```python
from build123d import *

# Parameters (mm, degrees)
SKETCH1_W                = 44.45
SKETCH1_H                = 57.15
SKETCH1_R                = 1.5875
BOSS_EXTRUDE1_DEPTH      = 1.5875
BOSS_EXTRUDE2_DEPTH      = 11.43
BOSS_EXTRUDE2_DEPTH_BACK = 3.81
BOSS_EXTRUDE3_REACH      = 120.467


with BuildPart() as part:
    # Sketch1 → Boss-Extrude1 (new body)
    with BuildSketch(Plane(origin=(0, 0, 0), x_dir=(1, 0, 0), z_dir=(0, 1, 0))):
        with Locations((-61.695053498, -38.539128831)):
            Rectangle(SKETCH1_W, SKETCH1_H)
        with Locations(Location((-80.745053498, -63.939128831, 0), (0, 0, 270))):
            Circle(SKETCH1_R, mode=Mode.SUBTRACT)
        with Locations(Location((-42.645053498, -63.939128831, 0), (0, 0, 270))):
            Circle(SKETCH1_R, mode=Mode.SUBTRACT)
        with Locations(Location((-42.645053498, -13.139128831, 0), (0, 0, 270))):
            Circle(SKETCH1_R, mode=Mode.SUBTRACT)
        with Locations(Location((-80.745053498, -13.139128831, 0), (0, 0, 270))):
            Circle(SKETCH1_R, mode=Mode.SUBTRACT)
    extrude(amount=BOSS_EXTRUDE1_DEPTH)

    # Sketch2 → Boss-Extrude2 (add, two sides: drawn at the far end of the back side and taken through both)
    with BuildSketch(Plane(origin=(0, 1.5875, 0), x_dir=(1, 0, 0), z_dir=(0, 1, 0)).offset(-BOSS_EXTRUDE2_DEPTH_BACK)):
        Polygon((-99.160053498, -6.789128831), (-83.920053498, -6.789128831), (-83.920053498, -70.289128831), (-99.160053498, -70.289128831), (-99.160053498, -69.394762634), (-86.755200336, -69.394762634), (-86.755200336, -64.028565451), (-99.160053498, -64.028565451), (-99.160053498, -63.134199254), (-86.755200336, -63.134199254), (-86.755200336, -57.768002071), (-99.160053498, -57.768002071), (-99.160053498, -56.873635873), (-86.755200336, -56.873635873), (-86.755200336, -51.50743869), (-99.160053498, -51.50743869), (-99.160053498, -50.613072493), (-86.755200336, -50.613072493), (-86.755200336, -45.24687531), (-99.160053498, -45.24687531), (-99.160053498, -44.352509113), (-86.755200336, -44.352509113), (-86.755200336, -38.98631193), (-99.160053498, -38.98631193), (-99.160053498, -38.091945732), (-86.755200336, -38.091945732), (-86.755200336, -32.725748549), (-99.160053498, -32.725748549), (-99.160053498, -31.831382352), (-86.755200336, -31.831382352), (-86.755200336, -26.465185169), (-99.160053498, -26.465185169), (-99.160053498, -25.570818972), (-86.755200336, -25.570818972), (-86.755200336, -20.204621789), (-99.160053498, -20.204621789), (-99.160053498, -19.310255592), (-86.755200336, -19.310255592), (-86.755200336, -13.944058409), (-99.160053498, -13.944058409), (-99.160053498, -13.049692211), (-86.755200336, -13.049692211), (-86.755200336, -7.683495028), (-99.160053498, -7.683495028), align=None)
        Polygon((-24.230053498, -7.683495028), (-24.230053498, -6.789128831), (-39.470053498, -6.789128831), (-39.470053498, -70.289128831), (-24.230053498, -70.289128831), (-24.230053498, -69.394762634), (-36.63490666, -69.394762634), (-36.63490666, -64.028565451), (-24.230053498, -64.028565451), (-24.230053498, -63.134199254), (-36.63490666, -63.134199254), (-36.63490666, -57.768002071), (-24.230053498, -57.768002071), (-24.230053498, -56.873635873), (-36.63490666, -56.873635873), (-36.63490666, -51.50743869), (-24.230053498, -51.50743869), (-24.230053498, -50.613072493), (-36.63490666, -50.613072493), (-36.63490666, -45.24687531), (-24.230053498, -45.24687531), (-24.230053498, -44.352509113), (-36.63490666, -44.352509113), (-36.63490666, -38.98631193), (-24.230053498, -38.98631193), (-24.230053498, -38.091945732), (-36.63490666, -38.091945732), (-36.63490666, -32.725748549), (-24.230053498, -32.725748549), (-24.230053498, -31.831382352), (-36.63490666, -31.831382352), (-36.63490666, -26.465185169), (-24.230053498, -26.465185169), (-24.230053498, -25.570818972), (-36.63490666, -25.570818972), (-36.63490666, -20.204621789), (-24.230053498, -20.204621789), (-24.230053498, -19.310255592), (-36.63490666, -19.310255592), (-36.63490666, -13.944058409), (-24.230053498, -13.944058409), (-24.230053498, -13.049692211), (-36.63490666, -13.049692211), (-36.63490666, -7.683495028), align=None)
    extrude(amount=BOSS_EXTRUDE2_DEPTH + BOSS_EXTRUDE2_DEPTH_BACK)

    # Boss-Extrude3: up to this face of the body (flat: up to its plane)
    boss_extrude3_end = Plane(part.part.faces().sort_by_distance((-91.540053498, 5.3975, 6.789128831))[0])
    # Sketch4 → Boss-Extrude3 (add, up to the picked face)
    with BuildSketch(Plane.XY.offset(70.289128831), mode=Mode.PRIVATE) as boss_extrude3_sk1:
        Polygon((-83.920053498, 0), (-82.920053498, 0), (-80.802621386, -1.2225), (-42.623870056, -1.2225), (-40.470053498, 0), (-39.470053498, 0), (-39.470053498, -1), (-40.206037044, -1), (-42.359853602, -2.2225), (-81.070570578, -2.2225), (-83.188002691, -1), (-83.920053498, -1), align=None)
    boss_extrude3_tool1 = split(extrude(boss_extrude3_sk1.sketch, amount=-BOSS_EXTRUDE3_REACH, mode=Mode.PRIVATE), bisect_by=boss_extrude3_end, keep=Keep.BOTH, mode=Mode.PRIVATE)
    add(boss_extrude3_tool1.solids().sort_by(Axis((-61.697362, -1.608795, 70.289129), (0, 0, -1)))[0])


solid = part.part
```
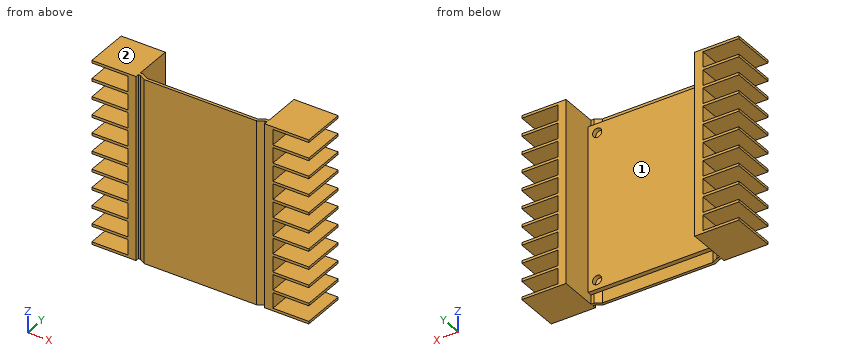
The model under review builds one solid part; all positions refer to its coordinate system, in mm. Face numbers are marked on the shaded views. A direction names the side the tool comes from. Round coordinates to 2 decimals unless told otherwise and drop trailing zeros. Write each loop counter-clockwise with the first axis right and the second up, starting at its lowest first coordinate (ties: lowest second). Pieces come first, ordered by that corner, then holes. Notation, with made-up numbers: (46.5, 40.5) - (79.5, 40.5) arc R13 cw to (79.5, 63.5) - close; hole circle Ø10 at (-13.5, 48). An arc over 180 degrees is marked (long way). Answer as CSV lines item,"result". Start each with the question number.
(1) For pin 1 Ø1.6 at (y, z) = (4.5, 48) entering from -X; pin 2 Ø2.5 at (y, z) = (6.5, 53) entering from +X; pin 3 Ø3 at (x, z) = (-75, 51.5) entering from +Y, all flat-tipped, find the tip position at first contact; note any pin that passes through.
(2) We need section A-A on x = -56. State the section outline as (y, z) points, plus the area to 3 significant figures.
(3) For the marked faces 1 and 2, list the 3-axis set-ups (+Z, -Z, +X, -X, +Y, -Y) from which the entire face can be reached by the end or side of a thin tool; tool diameter is ignored.
(4) We need section B-B on z = 60. State the section outline as (x, y) points, plus the area to 3 significant figures.
(5) To check wall thickness, follow line 1 (Y direction, x = -80, z = 54.5); line 2 (X direction, y = 9.25, z = 33); line 3 (X direction, y = 3.75, z = 32.5). State the ranges of each line that lie inside material, in increasing order.
(6) We need section C-C on x = -33.5. Give the number of separate pieces and of enclosed holes in the cut face, plus the area to 3 significant figures.
Worked answers:
1,pin 1,"x = -86.76"
1,pin 2,"x = -36.63"
1,pin 3,"y = 1.59"
2,outline,"(-2.22, 6.79) - (-1.22, 6.79) - (-1.22, 70.29) - (-2.22, 70.29) - close; (0, 9.96) - (1.59, 9.96) - (1.59, 67.11) - (0, 67.11) - close"
2,area,"154 mm²"
3,face 1,"+Z, -Z, +Y"
3,face 2,"+Z, +X, -X, +Y, -Y"
4,outline,"(-86.76, -2.22) - (-83.92, -2.22) - (-83.92, -1) - (-83.19, -1) - (-81.07, -2.22) - (-42.36, -2.22) - (-40.21, -1) - (-39.47, -1) - (-39.47, -2.22) - (-36.63, -2.22) - (-36.63, 13.02) - (-39.47, 13.02) - (-39.47, 1.59) - (-83.92, 1.59) - (-83.92, 13.02) - (-86.76, 13.02) - close; hole (-82.92, 0) - (-80.8, -1.22) - (-42.62, -1.22) - (-40.47, 0) - close"
4,area,"202 mm²"
5,line 1,"-2.22 to -1.22, 0 to 1.59"
5,line 2,"-86.76 to -83.92, -39.47 to -36.63"
5,line 3,"-99.16 to -83.92, -39.47 to -24.23"
6,separate pieces,"11"
6,enclosed holes,"0"
6,area,"150 mm²"
